Read the model definition and answer for the solid it produces. Units are mm, in the model's axes. Round coordinates to 2 decimals unless told otherwise and drop trailing zeros. Write each loop counter-clockwise with the first axis right and the second up, starting at its lowest first coordinate (ties: lowest second). Pieces come first, ordered by that corner, then holes. Notation, with made-up numbers: (-20.75, 54) - (-6.75, 54) arc R29 ccw to (-6.75, 86) - close; hole circle Ø2 at (-28, -16.5). An arc over 180 degrees is marked (long way). Use one line per item in the form item = value. Start each with the question number.
1) The part is cut by section C-C, the plane z = 29. Give the vertices of the cut face in (x, y).
2) The part is cut by section B-B, the plane x = 4.5. Count the separate pieces of the cut face and the enclosed holes in it, plus the area to 3 significant figures.
3) Consider line 1 along Z through (x, y) = (6.5, 5); line 2 along Z through (x, y) = (1.5, 4.75); line 3 along Y through (x, z) = (7, 3). Determine where each line is inside the solid, lowest interval first. Write a range as from..to.
4) The part is cut by section A-A, the plane z = 57. Give the vertices of the cut face in (x, y), plus the area to 3 significant figures.
5) Each of these flat-tipped pins is pushed along its axis until it touches: pin 1 (4 mm diameter, centred on x = 3.5, z = 30, fed in from -Y); pin 2 (4 mm diameter, centred on x = 3.5, y = 7.5, fed in from +Z); pin 3 (2 mm diameter, centred on x = 6, z = 29, fed in from +Y). Where does it stop, or does it pass through?
6) For a pull along Z with two mould halves and no side action, classify faces 1 (the face through (4.191, 10.797, 14.159)), 2 (the face through (4.19, 5.38, 58.6)), 3 (the face through (4.191, 20.364, 13.454)), 4 (the face through (4.2, 11.1, 7.9)) as released by +Z, released by -Z, zero draft, split by the parting line, or undercut.
from build123d import *

# Parameters (mm, degrees)
SKETCH1_R           = 1.749997696
SKETCH1_R_2         = 1.749993894
BOSS_EXTRUDE1_DEPTH = 8.500000462


with BuildPart() as part:
    # Sketch1 → Boss-Extrude1 (new body)
    with BuildSketch(Plane(origin=(0, 0, 0), x_dir=(0, -1, 0), z_dir=(-1, 0, 0))):
        Polygon((-0.127148596, 37.193398923), (-0.031888841, 37.750009447), (0, 38.313798606), (0, 60.313809663), (-0.03942649, 60.940481722), (-0.1570842, 61.557259411), (-0.351117604, 62.154430896), (-0.618466584, 62.722578645), (-0.954915013, 63.252732158), (-1.355157001, 63.736543059), (-1.812880044, 64.166367054), (-2.3208661, 64.535446465), (-2.87110405, 64.837940037), (-3.454915015, 65.06908685), (-4.063094035, 65.225243568), (-4.686047789, 65.303951502), (-5.313951988, 65.303951502), (-5.936907139, 65.225243568), (-6.545084994, 65.06908685), (-7.128897123, 64.837940037), (-7.679134142, 64.535446465), (-8.187118918, 64.166367054), (-8.644842543, 63.736543059), (-9.045084938, 63.252732158), (-9.3815336, 62.722578645), (-9.648882784, 62.154430896), (-9.842916392, 61.557259411), (-9.960573167, 60.940481722), (-9.999999776, 60.313809663), (-9.999999776, 51.61882937), (-10.003159754, 51.202278584), (-10.053309612, 49.896221608), (-10.166640393, 48.549070954), (-10.346939787, 47.150671482), (-10.599040426, 45.690581203), (-10.890450329, 44.321350753), (-11.248489842, 42.885411531), (-11.680469848, 41.3646698), (-12.197230011, 39.732418954), (-12.815520167, 37.947189063), (-13.558279723, 35.951770842), (-14.55048006, 33.42717886), (-15.819819644, 30.277069658), (-16.917720437, 27.492690831), (-17.711920664, 25.357909501), (-18.301250413, 23.649940267), (-18.799910322, 22.069010884), (-19.219560549, 20.58403939), (-19.567960873, 19.174400717), (-19.850589335, 17.825430259), (-20.071450621, 16.526099294), (-20.233500749, 15.267790295), (-20.338920876, 14.043499716), (-20.389260724, 12.84740027), (-20.385539159, 11.674479581), (-20.328279585, 10.52037999), (-20.217610523, 9.381227195), (-20.053209737, 8.253508247), (-19.83438991, 7.134027779), (-19.560100511, 6.019853055), (-19.228890538, 4.908256233), (-18.838969991, 3.796692938), (-18.388209864, 2.682805061), (-17.872419208, 1.56083703), (-14.189518528, -5.9e-07), (-11.067840271, 7.365807891), (-11.129870079, 8.45041126), (-11.15438994, 9.76248458), (-11.122629978, 11.049759574), (-11.035439558, 12.313780375), (-10.893439874, 13.556060381), (-10.697020218, 14.778049663), (-10.446329601, 15.981180593), (-10.141259991, 17.16681011), (-9.781503119, 18.3362104), (-9.366483428, 19.490620121), (-8.89539998, 20.6311699), (-8.367221802, 21.758910269), (-7.780684158, 22.874809802), (-7.134305779, 23.979740217), (-6.42638607, 25.074450299), (-5.655040033, 26.159580797), (-4.82408423, 27.228390798), (-0.502127572, 36.129970104), (-0.284564187, 36.651078612), align=None)
        with Locations((-5.001175624, 60.307227597)):
            Circle(SKETCH1_R, mode=Mode.SUBTRACT)
        with Locations((-5.000006282, 38.313804534)):
            Circle(SKETCH1_R_2, mode=Mode.SUBTRACT)
    extrude(amount=-BOSS_EXTRUDE1_DEPTH)


solid = part.part
Geometry results:
q1.outline = (0, 3.96) - (8.5, 3.96) - (8.5, 16.32) - (0, 16.32) - close
q2.separate_pieces = 1
q2.enclosed_holes = 2
q2.area = 635 mm2
q3.line_1 = 27..36.56, 40.06..58.56, 62.06..65.3
q3.line_2 = 27.38..36.58, 40.05..58.58, 62.04..65.3
q3.line_3 = 12.92..18.52
q4.outline = (0, 0) - (8.5, 0) - (8.5, 10) - (0, 10) - close
q4.area = 85.0 mm2
q5.pin_1 = 2.51
q5.pin_2 = 65.28
q5.pin_3 = 16.72
q6.face_1 = released by -Z
q6.face_2 = undercut
q6.face_3 = released by +Z
q6.face_4 = undercut
